Geometry: see drawing. Coordinates: mm, zero at the bounding-box minimum. Coordinates: 2 decimals unless noted, no trailing zeros. Order: outer loops, then holes, each group sorted by start corner. A loop starts at its lowest first (then second) coordinate and runs counter-clockwise, first axis right, second up. Notation, with made-up numbers: (3, -20.5) -> (17, -20.5) arc R14 ccw to (17, -10.5) -> close; hole circle Ø7 at (36.25, 21.5). An arc over 180 degrees is marked (long way). One line per item, written item: value. Start each with the question number.
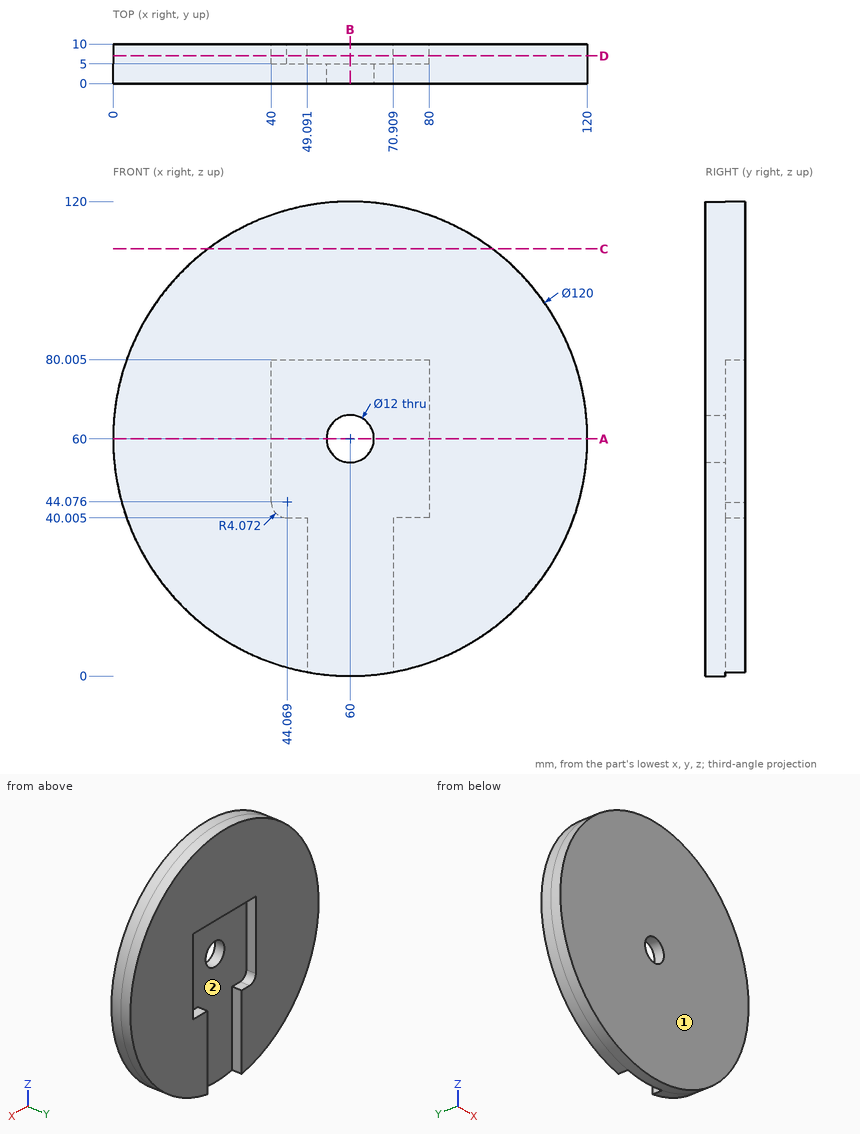
1) Mould query, pull axis X, two halves, no side actions, for the marked faces 1 and 2. Classes: +X half, -X half, draft (parallel to the pull), parting line (faces both ways), or undercut.
2) Section query C-C, the plane z = 108. Return the cut outline in (x, y), plus the area to 3 significant figures.
3) Section query D-D, the plane y = 7. Return the cut outline in (x, z) (1 decimal).
4) Ray query, line 1 along Z through (x, y) = (60, 1.95); line 2 along Y through (x, z) = (59.5, 35); line 3 along X through (y, z) = (9.25, 5). Return the intervals inside material, ascending. Write a range as from..to.
5) Pin query (flat end, axial travel): pin 1 Ø12 at (x, z) = (66.5, 48) entering from +Y; pin 2 Ø2.5 at (x, y) = (45.5, 8.5) entering from +Z; pin 3 Ø4 at (x, y) = (15, 8.5) entering from +Z (1 decimal). Return the tip coordinate at first contact, or that it passes through.
6) Section query A-A, the plane z = 60. Return the cut outline in (x, y).
7) Section query B-B, the plane x = 60. Return the cut outline in (y, z) (1 decimal).
Entries:
1. face 1: draft
1. face 2: undercut
2. outline: (24, 0) -> (96, 0) -> (96, 10) -> (24, 10) -> close
2. area: 720 mm2
3. outline: (40, 43.9) -> (40, 80) -> (80, 80) -> (80, 40) -> (70.9, 40) -> (70.9, 1) arc R60 ccw (long way) to (49.1, 1) -> (49.1, 40) -> (44, 40) arc R4.1 cw to start
4. line 1: z = 0..54, 66..120
4. line 2: y = 0..5
4. line 3: x = 36.02..49.09, 70.91..83.98
5. pin 1: stops at y = 5
5. pin 2: stops at z = 118.52
5. pin 3: stops at z = 101.8
6. outline: (0, 0) -> (54, 0) -> (54, 5) -> (40, 5) -> (40, 10) -> (0, 10) -> close; (66, 0) -> (120, 0) -> (120, 10) -> (80, 10) -> (80, 5) -> (66, 5) -> close
7. outline: (0, 0) -> (5, 0) -> (5, 54) -> (0, 54) -> close; (0, 66) -> (5, 66) -> (5, 80) -> (10, 80) -> (10, 120) -> (0, 120) -> close
